from build123d import *

# Parameters (mm, degrees)
SKETCH1_W           = 698.5
SKETCH1_H           = 254
SKETCH1_R           = 19.05
SKETCH1_R_2         = 9.525
BOSS_EXTRUDE1_DEPTH = 19.05
FILLET3_R           = 25.4
FILLET4_R           = 25.4
FILLET5_R           = 25.4
FILLET6_R           = 25.4
SKETCH2_R           = 19.05
BOSS_EXTRUDE2_DEPTH = 57.15


with BuildPart() as part:
    # Sketch1 → Boss-Extrude1 (new body)
    with BuildSketch(Plane.XY):
        Rectangle(SKETCH1_W, SKETCH1_H)
        with Locations(Location((0, 0, 0), (0, 0, 180))):
            Circle(SKETCH1_R, mode=Mode.SUBTRACT)
        with Locations(Location((-323.85, 101.6, 0), (0, 0, 180))):
            Circle(SKETCH1_R_2, mode=Mode.SUBTRACT)
        with Locations(Location((323.85, 101.6, 0), (0, 0, 180))):
            Circle(SKETCH1_R_2, mode=Mode.SUBTRACT)
        with Locations(Location((323.85, -101.6, 0), (0, 0, 180))):
            Circle(SKETCH1_R_2, mode=Mode.SUBTRACT)
        with Locations(Location((-323.85, -101.6, 0), (0, 0, 180))):
            Circle(SKETCH1_R_2, mode=Mode.SUBTRACT)
    extrude(amount=BOSS_EXTRUDE1_DEPTH)

    # Fillet3
    fillet3_edges = [part.edges().sort_by_distance(p)[0] for p in [
        (-349.25, 127, 9.525),
    ]]
    fillet(fillet3_edges, radius=FILLET3_R)

    # Fillet4
    fillet4_edges = [part.edges().sort_by_distance(p)[0] for p in [
        (-349.25, -127, 9.525),
    ]]
    fillet(fillet4_edges, radius=FILLET4_R)

    # Fillet5
    fillet5_edges = [part.edges().sort_by_distance(p)[0] for p in [
        (349.25, -127, 9.525),
    ]]
    fillet(fillet5_edges, radius=FILLET5_R)

    # Fillet6
    fillet6_edges = [part.edges().sort_by_distance(p)[0] for p in [
        (349.25, 127, 9.525),
    ]]
    fillet(fillet6_edges, radius=FILLET6_R)

    # Sketch2 → Boss-Extrude2 (add)
    with BuildSketch(Plane(origin=(349.25, 0, 0), x_dir=(0, 0, -1), z_dir=(1, 0, 0))):
        with BuildLine():
            Line((-19.05, 38.1), (-19.05, -38.1))
            Line((-19.05, -38.1), (-57.15, -38.1))
            ThreePointArc((-57.15, -38.1), (-95.25, 0), (-57.15, 38.1))
            Line((-57.15, 38.1), (-19.05, 38.1))
        make_face()
        with Locations((-57.15, 0)):
            Circle(SKETCH2_R, mode=Mode.SUBTRACT)
    boss_extrude2 = extrude(amount=-BOSS_EXTRUDE2_DEPTH)

    # Mirror3: Boss-Extrude2 across plane
    add(boss_extrude2.mirror(Plane.ZY))


solid = part.part
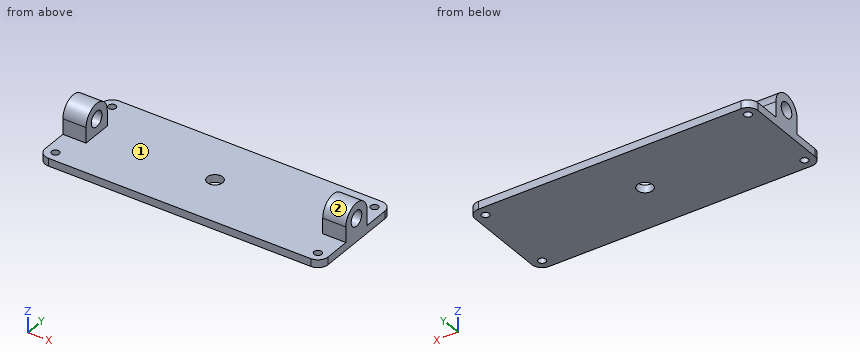
Here's how the part is built. I have some questions about the finished solid (model axes, mm). Face numbers are marked on the shaded views. Coordinates: 2 decimals unless noted, no trailing zeros. Write each loop counter-clockwise with the first axis right and the second up, starting at its lowest first coordinate (ties: lowest second). Pieces come first, ordered by that corner, then holes. Notation, with made-up numbers: (29.25, 1) - (37.25, 1) arc R16 cw to (37.25, 21) - close; hole circle Ø6 at (81.25, 44). An arc over 180 degrees is marked (long way). Use one line per item in the form item = value.
1) I need wall thicknesses on line 1 (X direction, y = -101, z = 11); line 2 (Y direction, x = 323, z = 8); line 3 (X direction, y = -4, z = 19.5). Which ranges of each line are inside material? Lowest first, please.
Solved:
line_1 = -349.25 to -333.36, -314.34 to 314.34, 333.36 to 349.25
line_2 = -127 to -111.09, -92.11 to 92.11, 111.09 to 127
line_3 = -349.25 to -292.1, 292.1 to 349.25
2) Thinking about a two-plate mould opening in X: for the marked faces 1 and 2, which applies, released by +X, released by -X, zero draft, split by the parting line, or undercut?
Solved:
face_1 = undercut
face_2 = zero draft
3) Suppose I cut it at D-D, the plane x = -98. Write out the boundary of the cut face in (y, z), plus the area to 3 significant figures.
Solved:
outline = (-127, 0) - (127, 0) - (127, 19.05) - (-127, 19.05) - close
area = 4,840 mm2
4) Suppose I cut it at A-A, the plane x = 0. Write out the boundary of the cut face in (y, z).
Solved:
outline = (-127, 0) - (-19.05, 0) - (-19.05, 19.05) - (-127, 19.05) - close; (19.05, 0) - (127, 0) - (127, 19.05) - (19.05, 19.05) - close
5) Suppose I cut it at C-C, the plane y = 50. Write out the boundary of the cut face in (x, z), plus the area to 3 significant figures.
Solved:
outline = (-349.25, 0) - (349.25, 0) - (349.25, 19.05) - (-349.25, 19.05) - close
area = 13,300 mm2
6) Suppose I cut it at B-B, the plane x = 305. Write out the boundary of the cut face in (y, z).
Solved:
outline = (-127, 0) - (127, 0) - (127, 19.05) - (38.1, 19.05) - (38.1, 57.15) arc R38.1 ccw to (-38.1, 57.15) - (-38.1, 19.05) - (-127, 19.05) - close; hole circle Ø38.1 at (0, 57.15)
7) I'm going to push flat-ended pins straight in: P1, Ø2, axis at x = 107.5, y = -90, coming from the -Z side; P2, Ø25, axis at x = -323.85, y = 101.6, coming from the +Z side; P3, Ø19, axis at x = 333, z = 46, coming from the -Y side. Where does each tip first touch, or does it pass through?
Solved:
P1 = 0
P2 = 19.05
P3 = -38.1
